Part print with two shaded views. Sizes in mm from the minimum x, y, z corner. Round coordinates to 2 decimals unless told otherwise and drop trailing zeros. Write each loop counter-clockwise with the first axis right and the second up, starting at its lowest first coordinate (ties: lowest second). Pieces come first, ordered by that corner, then holes. Notation, with made-up numbers: (-33.5, 4.25) -> (5.5, 4.25) arc R18 ccw to (5.5, 30.25) -> close; hole circle Ø5 at (2.5, 41.5). An arc over 180 degrees is marked (long way). Put each result on its own line as item: value. Start each with the question number.
1. Flat gauge pin, fed straight in: P1, Ø1.5, axis at x = 56, z = 62, coming from the -Y side. Where does the tip first touch, or does it go through?
2. Saw through at D-D on x = 23.5. List the corners of the cut face in (y, z).
3. Drill centre lines: line 1 (X direction, y = 2.5, z = 62); line 2 (Z direction, x = 20, y = 3); line 3 (Y direction, x = 56, z = 31). Where is each one in solid material? Low to high. Write a range as from..to.
4. Pull direction X, two halves, no side cores. Call the marked faces 1 and 2: pulls with the +X half, pulls with the -X half, needs draft (parallel to the pull), parting line crosses it, or undercut.
5. Saw through at B-B on z = 128.5. List the corners of the cut face in (x, y) (1 decimal), and give its area (3 significant figures).
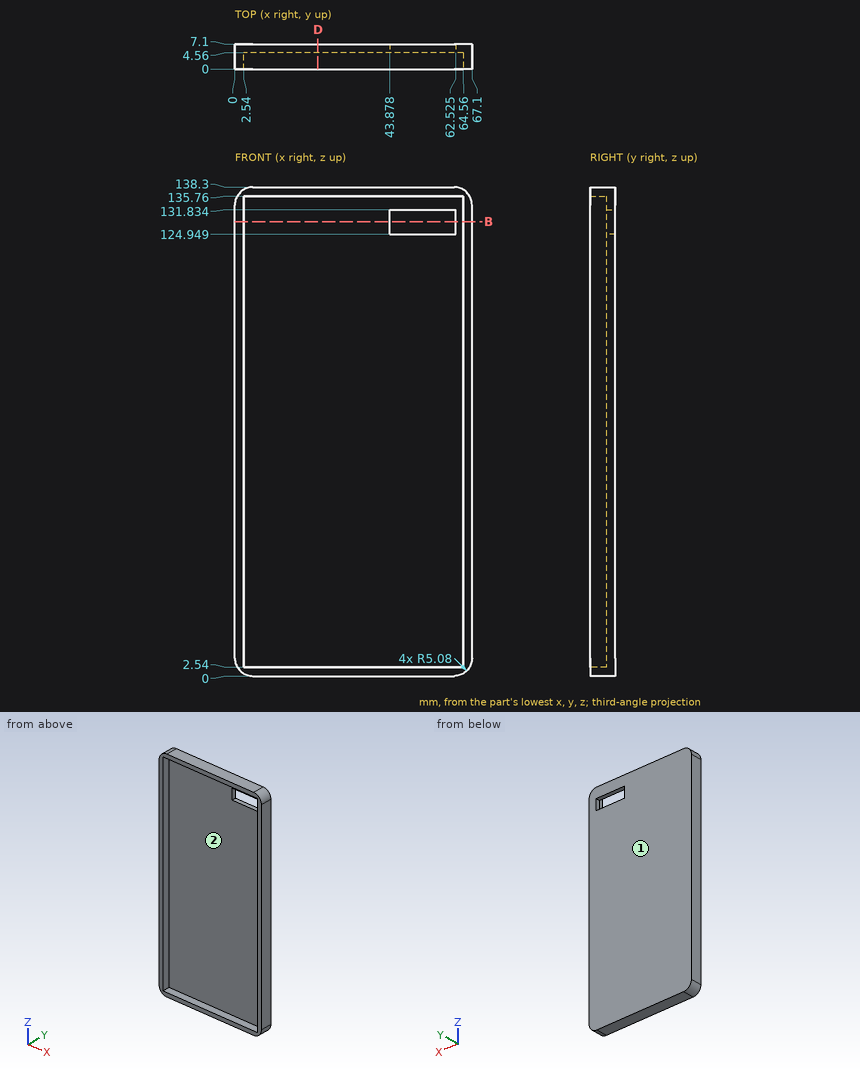
Return value:
1. P1: stops at y = 4.56
2. outline: (0, 0) -> (7.1, 0) -> (7.1, 138.3) -> (0, 138.3) -> (0, 135.76) -> (4.56, 135.76) -> (4.56, 2.54) -> (0, 2.54) -> close
3. line 1: x = 0..2.54, 64.56..67.1
3. line 2: z = 0..2.54, 135.76..138.3
3. line 3: y = 4.56..7.1
4. face 1: needs draft
4. face 2: undercut
5. outline: (0, 0) -> (2.5, 0) -> (2.5, 4.6) -> (43.9, 4.6) -> (43.9, 7.1) -> (0, 7.1) -> close; (62.5, 4.6) -> (64.6, 4.6) -> (64.6, 0) -> (67.1, 0) -> (67.1, 7.1) -> (62.5, 7.1) -> close
5. area: 146 mm^2
